```python
from build123d import *

# Parameters (mm, degrees)
F0_R     = 7.874
F1_DEPTH = 152.4
F2_R     = 15.875
F3_DEPTH = 173.736
F5_DEPTH = 186.436


with BuildPart() as f1:
    # F0 (on Top) → F1 (new body)
    with BuildSketch(Plane.XY):
        Polygon((0, 50.8), (0, 0), (133.096, 0), (133.096, 50.8), (66.548, 50.8), align=None)
        with Locations((18.796, 25.4)):
            Circle(F0_R, mode=Mode.SUBTRACT)
        with Locations((114.3, 25.4)):
            Circle(F0_R, mode=Mode.SUBTRACT)
    extrude(amount=F1_DEPTH)

    # F2 (on face) → F3 (cut)
    with BuildSketch(Plane.XZ):
        with BuildLine():
            Line((0, 152.4), (0, 12.7))
            Line((0, 12.7), (38.1, 12.7))
            Line((38.1, 12.7), (38.1, 15.748))
            Line((38.1, 15.748), (38.1, 41.148))
            ThreePointArc((38.1, 41.148), (66.548, 69.596), (94.996, 41.148))
            Line((94.996, 41.148), (94.996, 15.748))
            Line((94.996, 15.748), (94.996, 12.7))
            Line((94.996, 12.7), (133.096, 12.7))
            Line((133.096, 12.7), (133.096, 152.4))
            Line((133.096, 152.4), (0, 152.4))
        make_face()
        with Locations((66.548, 41.148)):
            Circle(F2_R)
    extrude(amount=-F3_DEPTH, mode=Mode.SUBTRACT)

    # F4 (on Right) → F5 (cut)
    with BuildSketch(Plane.YZ):
        Polygon((0, 77.27585), (0, 15.748), (22.439078, 77.39886), align=None)
    extrude(amount=F5_DEPTH, mode=Mode.SUBTRACT)


solid = f1.part
```
Can you work these out from the model? Positions are in its coordinate system, mm. A direction names the side the tool comes from. Coordinates: 2 decimals unless noted, no trailing zeros. Loops run counter-clockwise (first coordinate to the right, second up) from the corner with the lowest first, then second, coordinate; pieces in that order, holes last.
1) Thinking about a two-plate mould opening in X: for faces 4 (the cylindrical face through (106.434, 25.746, 6.261)), 5 (the flat face through (133.096, 25, 6)), 6 (the cylindrical face through (65.92, 34.35, 69.59)), 7 (the flat face through (105, 25, 12.7)), which applies, pulls with the +X half, pulls with the -X half, needs draft (parallel to the pull), parting line crosses it, or undercut?
2) Imagine slicing it at A-A on y = 25.4. List the corners of the cut face in (x, z) for me (3 decimals).
3) Imagine slicing it at C-C on z = 8.5. List the corners of the cut face in (x, y) for me.
4) Which directions (+Z, -Z, +X, -X, +Y, -Y) give clear straight access to the entire face, cutting with the end or side of a thin tool? Please do faces 1 (the flat face through (66, 26, 0)), 2 (the flat face through (94.996, 25, 27)), 3 (the flat face through (38.1, 25, 27)).
5) I need wall thicknesses on probe 1 along X at (y, z) = (25.4, 9.5); probe 2 along Y at (x, z) = (114.3, 2.5); probe 3 along X at (y, z) = (31.5, 12.5). Which ranges of each line are inside material? Lowest first, please.
6) Imagine slicing it at B-B on x = 114.3. List the corners of the cut face in (y, z) for me, plus the area to 3 significant figures.
7) For pin 1 (8 mm diameter, centred on y = 8, z = 24.5, fed in from -X); pin 2 (5 mm diameter, centred on x = 58, y = 23, fed in from +Z); pin 3 (5 mm diameter, centred on x = 33.5, y = 12, fed in from +Z), each with a flat end and sliding along its axis, tell me the tip position at first contact or that it passes through.
8) Imagine slicing it at D-D on z = 28.5. List the corners of the cut face in (x, y) for me.
Completed:
1. face 4: undercut
1. face 5: pulls with the +X half
1. face 6: parting line crosses it
1. face 7: needs draft
2. outline: (0, 0) - (10.922, 0) - (10.922, 12.7) - (0, 12.7) - close; (26.67, 0) - (106.426, 0) - (106.426, 12.7) - (94.996, 12.7) - (94.996, 41.148) arc R28.448 ccw to (38.1, 41.148) - (38.1, 12.7) - (26.67, 12.7) - close; (122.174, 0) - (133.096, 0) - (133.096, 12.7) - (122.174, 12.7) - close; hole circle Ø31.75 at (66.548, 41.148)
3. outline: (0, 0) - (133.1, 0) - (133.1, 50.8) - (0, 50.8) - close; hole circle Ø15.75 at (18.8, 25.4); hole circle Ø15.75 at (114.3, 25.4)
4. face 1: -Z, +X, -X, +Y, -Y
4. face 2: +Z, +X, +Y, -Y
4. face 3: +Z, -X, +Y, -Y
5. probe 1: x = 0 to 10.92, 26.67 to 106.43, 122.17 to 133.1
5. probe 2: y = 0 to 17.53, 33.27 to 50.8
5. probe 3: x = 0 to 13.82, 23.77 to 109.32, 119.28 to 133.1
6. outline: (0, 0) - (17.53, 0) - (17.53, 12.7) - (0, 12.7) - close; (33.27, 0) - (50.8, 0) - (50.8, 12.7) - (33.27, 12.7) - close
6. area: 445 mm2
7. pin 1: stops at x = 38.1
7. pin 2: stops at z = 68.95
7. pin 3: stops at z = 12.7
8. outline: (38.1, 4.64) - (56.95, 4.64) - (56.95, 50.8) - (38.1, 50.8) - close; (76.14, 4.64) - (95, 4.64) - (95, 50.8) - (76.14, 50.8) - close
